Read the model definition and answer for the solid it produces. Units are mm, in the model's axes. A direction names the side the tool comes from. Round coordinates to 2 decimals unless told otherwise and drop trailing zeros. Loops run counter-clockwise (first coordinate to the right, second up) from the corner with the lowest first, then second, coordinate; pieces in that order, holes last. Notation, with made-up numbers: M 81.25,-40 L 136.25,-40 A20 cw 136.25,-12 Z; hole C -18.5,14 d5. An arc over 180 degrees is marked long. Answer as CSV lines item,"result".
```python
from build123d import *

# Parameters (mm, degrees)
SKETCH_1_R      = 2
SKETCH_1_R_2    = 1.55
SKETCH_1_R_3    = 1.25
SKETCH_1_W      = 10
SKETCH_1_H      = 6.1
EXTRUDE_1_DEPTH = 6


with BuildPart() as part:
    # Эскиз1 → Бобышка-Вытянуть1 (new body)
    with BuildSketch(Plane.XY):
        with BuildLine():
            Line((160, 156), (160, 136))
            ThreePointArc((160, 136), (149.118825479, 0), (160, -136))
            Line((160, -136), (160, -156))
            ThreePointArc((160, -156), (158.828427125, -158.828427125), (156, -160))
            Line((156, -160), (136, -160))
            Line((136, -160), (-156, -160))
            ThreePointArc((-156, -160), (-158.828427125, -158.828427125), (-160, -156))
            Line((-160, -156), (-160, -136))
            ThreePointArc((-160, -136), (-149.118825479, 0), (-160, 136))
            Line((-160, 136), (-160, 156))
            ThreePointArc((-160, 156), (-158.828427125, 158.828427125), (-156, 160))
            Line((-156, 160), (136, 160))
            Line((136, 160), (156, 160))
            ThreePointArc((156, 160), (158.828427125, 158.828427125), (160, 156))
        make_face()
        with Locations((-154.5, 154)):
            Circle(SKETCH_1_R, mode=Mode.SUBTRACT)
        with Locations((-154.5, -154)):
            Circle(SKETCH_1_R, mode=Mode.SUBTRACT)
        with Locations((154.5, 154)):
            Circle(SKETCH_1_R, mode=Mode.SUBTRACT)
        with Locations((154.5, -154)):
            Circle(SKETCH_1_R, mode=Mode.SUBTRACT)
        with Locations((117.1, -123.55)):
            Circle(SKETCH_1_R_2, mode=Mode.SUBTRACT)
        with Locations((-117.1, -123.55)):
            Circle(SKETCH_1_R_2, mode=Mode.SUBTRACT)
        with Locations((-117.1, 123.55)):
            Circle(SKETCH_1_R_2, mode=Mode.SUBTRACT)
        with Locations((117.1, 123.55)):
            Circle(SKETCH_1_R_2, mode=Mode.SUBTRACT)
        with Locations((142.88852833, -154.406847052)):
            Circle(SKETCH_1_R_3, mode=Mode.SUBTRACT)
        with Locations((137.91717333, -154.338989052)):
            Circle(SKETCH_1_R_3, mode=Mode.SUBTRACT)
        with Locations((-0.5, 154)):
            Circle(SKETCH_1_R, mode=Mode.SUBTRACT)
        with Locations((144.264881547, 152.244611453)):
            Circle(SKETCH_1_R_3, mode=Mode.SUBTRACT)
        with Locations((139.293526547, 152.312469453)):
            Circle(SKETCH_1_R_3, mode=Mode.SUBTRACT)
        with Locations((97.1, 123.55)):
            Rectangle(SKETCH_1_W, SKETCH_1_H, mode=Mode.SUBTRACT)
        with Locations((-97.1, -123.55)):
            Rectangle(SKETCH_1_W, SKETCH_1_H, mode=Mode.SUBTRACT)
        with Locations((97.1, -123.55)):
            Rectangle(SKETCH_1_W, SKETCH_1_H, mode=Mode.SUBTRACT)
        with Locations((-97.1, 123.55)):
            Rectangle(SKETCH_1_W, SKETCH_1_H, mode=Mode.SUBTRACT)
        with BuildLine():
            Line((93.489652385, -94.205074627), (2.780610095, -20.466408797))
            ThreePointArc((2.780610095, -20.466408797), (-1.333842507, -18.299575929), (-5.45296535, -20.457517519))
            Line((-5.45296535, -20.457517519), (-96.398158259, -94.197961604))
            ThreePointArc((-96.398158259, -94.197961604), (-96.649394743, -98.329753251), (-93.107179505, -100.471606))
            Line((-93.107179505, -100.471606), (90.193770783, -100.471606))
            ThreePointArc((90.193770783, -100.471606), (93.73397738, -98.333577335), (93.489652385, -94.205074627))
        make_face(mode=Mode.SUBTRACT)
        with BuildLine():
            Line((-5.393845546, 20.503538093), (-96.102893823, 94.242212627))
            ThreePointArc((-96.102893823, 94.242212627), (-96.347218817, 98.370715335), (-92.807012221, 100.508744))
            Line((-92.807012221, 100.508744), (90.493950067, 100.508744))
            ThreePointArc((90.493950067, 100.508744), (94.036165305, 98.366891251), (93.784928821, 94.235099604))
            Line((93.784928821, 94.235099604), (2.839729898, 20.494646814))
            ThreePointArc((2.839729898, 20.494646814), (-1.279392944, 18.336705225), (-5.393845546, 20.503538093))
        make_face(mode=Mode.SUBTRACT)
        with BuildLine():
            Line((-109.763358937, -84.575917132), (-13.303284143, -2.757613876))
            ThreePointArc((-13.303284143, -2.757613876), (-12.418558312, 0.078161869), (-13.298704681, 2.915362292))
            Line((-13.298704681, 2.915362292), (-109.49916318, 84.639383129))
            ThreePointArc((-109.49916318, 84.639383129), (-116.218458744, 86.97087694), (-120.442977971, 81.249143499))
            Line((-120.442977971, 81.249143499), (-120.701678374, -81.158585361))
            ThreePointArc((-120.701678374, -81.158585361), (-116.49090996, -86.895155762), (-109.763358937, -84.575917132))
        make_face(mode=Mode.SUBTRACT)
        with BuildLine():
            Line((106.88592289, -84.602246797), (10.646219109, -2.821157348))
            ThreePointArc((10.646219109, -2.821157348), (9.766074027, 0.017406269), (10.652347669, 2.854062364))
            Line((10.652347669, 2.854062364), (107.15201684, 84.634313992))
            ThreePointArc((107.15201684, 84.634313992), (113.879270457, 86.95037229), (118.088477358, 81.21428961))
            Line((118.088477358, 81.21428961), (117.82973768, -81.212007525))
            ThreePointArc((117.82973768, -81.212007525), (113.605218283, -86.933740662), (106.88592289, -84.602246797))
        make_face(mode=Mode.SUBTRACT)
    extrude(amount=EXTRUDE_1_DEPTH)


solid = part.part
```
1) Straight lines are drawn through the part: line 1 (X direction, y = 46.5, z = 1.25); line 2 (X direction, y = -47, z = 5.3); line 3 (Y direction, x = -117.1, z = 2.1). For each, find the intervals that lie inside material, in ascending order.
Evaluation:
line 1,"x = -150.38 to -120.5, -64.6 to -37.37, 34.91 to 62.15, 118.03 to 150.38"
line 2,"x = -150.41 to -120.65, -65.46 to -38.19, 35.42 to 62.64, 117.88 to 150.41"
line 3,"y = -160 to -125.1, -122 to -86.67, 86.62 to 122, 125.1 to 160"
2) This flat-tipped pin is pushed along its axis until it touches: P1, Ø2.5, axis at x = -154.5, y = -154, coming from the -Z side. Where does it stop, or does it pass through?
Evaluation:
P1,"passes through"
3) Find section D-D, the plane z = 2.45. Count the separate pieces of the cut face and the enclosed holes in it, then the cut area to 3 significant figures.
Evaluation:
separate pieces,"1"
enclosed holes,"21"
area,"60,400 mm^2"
4) Find section C-C, the plane y = -11.5. Give the vertices of the cut face in (x, z).
Evaluation:
outline,"M -149.2,0 L -120.59,0 L -120.59,6 L -149.2,6 Z; M -23.61,0 L 20.86,0 L 20.86,6 L -23.61,6 Z; M 117.94,0 L 149.2,0 L 149.2,6 L 117.94,6 Z"
5) Find section B-B, the plane y = 43. Give the vertices of the cut face in (x, z), then the cut area to 3 significant figures.
Evaluation:
outline,"M -150.2,0 L -120.5,0 L -120.5,6 L -150.2,6 Z; M -60.48,0 L -33.07,0 L -33.07,6 L -60.48,6 Z; M 30.6,0 L 58.02,0 L 58.02,6 L 30.6,6 Z; M 118.03,0 L 150.2,0 L 150.2,6 L 118.03,6 Z"
area,"700 mm^2"
6) Find section A-A, the plane x = -67. Give the vertices of the cut face in (y, z), then the cut area to 3 significant figures.
Evaluation:
outline,"M -160,0 L -100.47,0 L -100.47,6 L -160,6 Z; M -70.36,0 L -48.3,0 L -48.3,6 L -70.36,6 Z; M 48.54,0 L 70.58,0 L 70.58,6 L 48.54,6 Z; M 100.51,0 L 160,0 L 160,6 L 100.51,6 Z"
area,"979 mm^2"
7) Determine the mould class of faces 3 (the flat face through (-50.113, 56.857, 2.958)), 4 (the cylindrical face through (-149.12, -1.91, 2.96)), 5 (the flat face through (2, 2, 6)), 6 (the flat face through (58.227, 43.172, 2.958)) for opening direction X: released by +X, released by -X, zero draft, split by the parting line, or undercut.
Evaluation:
face 3,"undercut"
face 4,"released by -X"
face 5,"zero draft"
face 6,"undercut"
8) A tool of negligible diameter and unlimited length cuts with its end or side. For faces 1 (the flat face through (-60.73, 43.21, 2.96)), 2 (the flat face through (2, 2, 0)), from which of +Z, -Z, +X, -X, +Y, -Y can it reach the whole face along a straight path? Write none if from no direction.
Evaluation:
face 1,"+Z, -Z"
face 2,"-Z, +X, -X, +Y, -Y"
